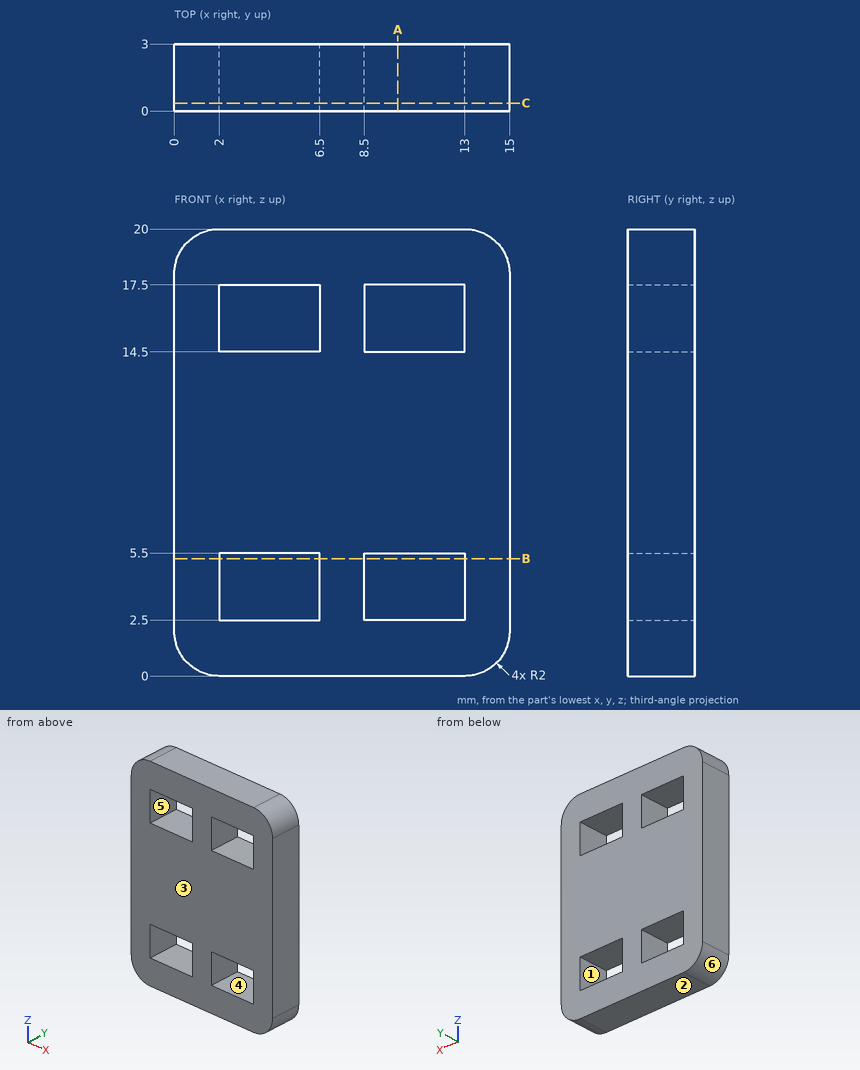
Study the drawing (mm; zero at the part's minimum x, y, z) and answer. A direction names the side the tool comes from. Round coordinates to 2 decimals unless told otherwise and drop trailing zeros. Loops run counter-clockwise (first coordinate to the right, second up) from the corner with the lowest first, then second, coordinate; pieces in that order, holes last.
Q1. Find the intervals of material crossed by line 1 (X direction, y = 0.35, z = 15); line 2 (Z direction, x = 9.5, y = 1.2); line 3 (Z direction, x = 14, y = 0.35), in increasing order.
Q2. For a pull along Z with two mould halves and no side action, classify the marked faces 3, 4, 5 and 6 as released by +Z, released by -Z, zero draft, split by the parting line, or undercut.
Q3. Section A-A, the plane x = 10 is taken. Determine the outline of the cut face in (y, z).
Q4. Which of the six approach directions +Z, -Z, +X, -X, +Y, -Y give full straight-line access (tool end or side, diameter ignored) to the marked faces 1 and 2?
Q5. Section B-B, the plane z = 5.25 is taken. Determine the outline of the cut face in (x, y), then the cut area to 3 significant figures.
Q6. Section C-C, the plane y = 0.35 is taken. Determine the outline of the cut face in (x, z), then the cut area to 3 significant figures.
Completed:
1. line 1: x = 0 to 2, 6.5 to 8.5, 13 to 15
1. line 2: z = 0 to 2.5, 5.5 to 14.5, 17.5 to 20
1. line 3: z = 0.27 to 19.73
2. face 3: zero draft
2. face 4: undercut
2. face 5: undercut
2. face 6: released by -Z
3. outline: (0, 0) - (3, 0) - (3, 2.5) - (0, 2.5) - close; (0, 5.5) - (3, 5.5) - (3, 14.5) - (0, 14.5) - close; (0, 17.5) - (3, 17.5) - (3, 20) - (0, 20) - close
4. face 1: +Y, -Y
4. face 2: -Z, +X, -X, +Y, -Y
5. outline: (0, 0) - (2, 0) - (2, 3) - (0, 3) - close; (6.5, 0) - (8.5, 0) - (8.5, 3) - (6.5, 3) - close; (13, 0) - (15, 0) - (15, 3) - (13, 3) - close
5. area: 18.0 mm2
6. outline: (0, 2) arc R2 ccw to (2, 0) - (13, 0) arc R2 ccw to (15, 2) - (15, 18) arc R2 ccw to (13, 20) - (2, 20) arc R2 ccw to (0, 18) - close; hole (2, 2.5) - (6.5, 2.5) - (6.5, 5.5) - (2, 5.5) - close; hole (2, 14.5) - (6.5, 14.5) - (6.5, 17.5) - (2, 17.5) - close; hole (8.5, 2.5) - (13, 2.5) - (13, 5.5) - (8.5, 5.5) - close; hole (8.5, 14.5) - (13, 14.5) - (13, 17.5) - (8.5, 17.5) - close
6. area: 243 mm2
